```python
from build123d import *

# Parameters (mm, degrees)
F3_DEPTH = 4
F4_SIZE  = 4.99999


# Not quite as in the source:
# - a fillet or chamfer is up to 0.001 mm smaller than in the source, because OpenCascade refuses the exact size


with BuildPart() as f1:
    # F0 (on Front) → F1 (revolve)
    with BuildSketch(Plane.XZ):
        Polygon((5.5, 5), (5.5, 10), (0, 10), (0, 0), (50, 0), (50, 4.25), (49.25, 5), (8.5, 5), (8.375, 4.25), (8.25, 5), align=None)
    revolve(axis=Axis((25, 0, 0), (1, 0, 0)))

    # F2 (on face) → F3 (cut)
    with BuildSketch(Plane(origin=(0, 0, 0), x_dir=(0, -1, 0), z_dir=(-1, 0, 0))):
        Polygon((0, -2.8867513459), (2.5, -1.443375673), (2.5, 1.443375673), (0, 2.8867513459), (-2.5, 1.443375673), (-2.5, -1.443375673), align=None)
    extrude(amount=-F3_DEPTH, mode=Mode.SUBTRACT)

    # F4 (size 5 in the source; OpenCascade refuses exactly that, so slightly less here)
    f4_edges = [f1.edges().sort_by_distance(p)[0] for p in [
        (5.5, 0, -10),
    ]]
    chamfer(f4_edges, length=F4_SIZE)


solid = f1.part
```
Input: part model. Units: mm. Frame: model coordinates. A direction names the side the tool comes from. Round coordinates to 2 decimals unless told otherwise and drop trailing zeros. Loops run counter-clockwise (first coordinate to the right, second up) from the corner with the lowest first, then second, coordinate; pieces in that order, holes last.
1) Section query B-B on x = 20.5. Return the cut outline in (y, z).
Ans:
outline: circle Ø10 at (0, 0)
2) Pin query (flat end, axial travel): pin 1 (5 mm diameter, centred on x = 22, y = 0, fed in from -Z); pin 2 (1 mm diameter, centred on x = 23, y = -7, fed in from +Z) (3 decimals); pin 3 (1.5 mm diameter, centred on y = 0, z = 0.5, fed in from -X); pin 4 (2.5 mm diameter, centred on x = 2.5, z = 0.5, fed in from -Y). Return the tip coordinate at first contact, or that it passes through.
Ans:
pin 1: stops at z = -5
pin 2: passes through
pin 3: stops at x = 4
pin 4: stops at y = -9.24
3) Material intervals for line 1 (X direction, y = 1.75, z = 6); line 2 (Z direction, x = 26.5, y = 2.5); line 3 (X direction, y = 4.75, z = -6), sorted ascending.
Ans:
line 1: x = 0 to 4.25
line 2: z = -4.33 to 4.33
line 3: x = 0 to 2.85
4) Set-up query: faces 4 (the cylindrical face through (28.59, 4.88, -1.08)), 5 (the flat face through (2, -2.5, 0)), 6 (the cylindrical face through (0.25, 9.76, -2.17)). Return all of +Z, -Z, +X, -X, +Y, -Y with unobstructed straight access to the full face (end or side cutting, diameter ignored); none if empty.
Ans:
face 4: +X
face 5: -X
face 6: +X, -X
5) Pull-direction query (Y, two-part tool) for faces 1 (the cylindrical face through (6.86, 4.88, -1.08)), 2 (the flat face through (2, 2.5, 0)), 3 (the flat face through (50, 0, 0)); classes: released by +Y, released by -Y, zero draft, split by the parting line, or undercut.
Ans:
face 1: split by the parting line
face 2: undercut
face 3: zero draft
